Geometry check sheet. Reference: the model listing, model coordinates, mm. A direction names the side the tool comes from. Round coordinates to 2 decimals unless told otherwise and drop trailing zeros. Loops run counter-clockwise (first coordinate to the right, second up) from the corner with the lowest first, then second, coordinate; pieces in that order, holes last. Notation, with made-up numbers: M 71,52 L 75,52 A13 cw 75,63 Z; hole C 68,77 d10. An arc over 180 degrees is marked long. Write item = value, one per line.
from build123d import *

# Parameters (mm, degrees)
F0_R     = 3
F1_DEPTH = 5
F3_DEPTH = 115
F5_DEPTH = 25
F7_DEPTH = 25


with BuildPart() as f1:
    # F0 (on Top) → F1 (new body)
    with BuildSketch(Plane.XY):
        Polygon((-74.838845, -4.279941), (-74.838845, -104.279941), (35.161155, -104.279941), (35.161155, -4.279941), (30.161155, -4.279941), (30.161155, -39.279941), (-69.838845, -39.279941), (-69.838845, -4.279941), align=None)
        with Locations((-49.838845, -54.279941)):
            Circle(F0_R, mode=Mode.SUBTRACT)
        with Locations((10.161155, -54.279941)):
            Circle(F0_R, mode=Mode.SUBTRACT)
    extrude(amount=F1_DEPTH)

    # F2 (on face) → F3 (join)
    with BuildSketch(Plane.XY.offset(5)):
        Polygon((-74.838845, -104.279941), (-69.838845, -104.279941), (-69.838845, -39.279941), (-69.838845, -4.279941), (-74.838845, -4.279941), align=None)
        Polygon((30.161155, -39.279941), (30.161155, -104.279941), (35.161155, -104.279941), (35.161155, -4.279941), (30.161155, -4.279941), align=None)
    extrude(amount=F3_DEPTH)

    # F4 (on face) → F5 (cut)
    with BuildSketch(Plane.YZ.offset(35.161155)):
        Polygon((-104.279941, 30), (-34.279941, 120), (-104.279941, 120), align=None)
        with BuildLine():
            Line((-4.279941, 100), (-4.279941, 109.995835))
            Line((-4.279941, 109.995835), (-14.075894, 109.995835))
            Line((-14.075894, 109.995835), (-14.483987, 109.995835))
            ThreePointArc((-14.483987, 109.995835), (-19.2789, 104.897956), (-14.279941, 100))
            Line((-14.279941, 100), (-4.279941, 100))
        make_face()
    extrude(amount=-F5_DEPTH, mode=Mode.SUBTRACT)

    # F6 (on face) → F7 (cut)
    with BuildSketch(Plane(origin=(-74.838845, 0, 0), x_dir=(0, -1, 0), z_dir=(-1, 0, 0))):
        with BuildLine():
            Line((13.948806, 109.989023), (4.279941, 109.989023))
            Line((4.279941, 109.989023), (4.279941, 100))
            Line((4.279941, 100), (14.279941, 100))
            ThreePointArc((14.279941, 100), (19.277196, 104.834341), (14.611076, 109.989023))
            Line((14.611076, 109.989023), (13.948806, 109.989023))
        make_face()
        Polygon((104.279941, 120), (34.279941, 120), (104.279941, 30), align=None)
    extrude(amount=-F7_DEPTH, mode=Mode.SUBTRACT)


solid = f1.part
(1) Tool access check on faces 1 (the flat face through (33, -9, 109.996)), 2 (the flat face through (33, -4.28, 115)), 3 (the flat face through (-21, -71, 5)). Record the directions out of +Z, -Z, +X, -X, +Y, -Y that give a thin tool (end or side, any length) a straight path to the whole face; none if there is none.
Result set:
face_1 = +X, -X, +Y
face_2 = +Z, -Z, +X, -X, +Y
face_3 = +Z, +Y, -Y
(2) Depth check by flat-ended pin: pin 1 Ø19.5 at (x, y) = (0.5, -56.5) entering from +Z; pin 2 Ø2.5 at (x, z) = (-20.5, 2.5) entering from +Y; pin 3 Ø5.5 at (x, y) = (10.16, -54.28) entering from +Z. Enter the tip coordinate at first touch or a pass-through.
Result set:
pin_1 = 5
pin_2 = -39.28
pin_3 = through
(3) Sectioned sample at C-C on x = 18. Record the cut outline in (y, z).
Result set:
outline = M -104.28,0 L -39.28,0 L -39.28,5 L -104.28,5 Z
(4) Material ranges on line 1 along X through (y, z) = (-51, 51); line 2 along Z through (x, y) = (-2, -55), recorded low to high. Write a range as from..to.
Result set:
line_1 = -74.84..-69.84, 30.16..35.16
line_2 = 0..5
(5) Sectioned sample at D-D on y = -77. Record the cut outline in (x, z).
Result set:
outline = M -74.84,0 L 35.16,0 L 35.16,65.07 L 30.16,65.07 L 30.16,5 L -69.84,5 L -69.84,65.07 L -74.84,65.07 Z
(6) Release check for a two-part mould opening along X. For faces 4 (the cylindrical face through (9.51, -57.21, 2.46)), 5 (the flat face through (-72, -4.28, 115)), 6 (the flat face through (-19, -39.28, 2)), 7 (the flat face through (35.161, -44, 46)) record: released by +X, released by -X, zero draft, split by the parting line, or undercut.
Result set:
face_4 = undercut
face_5 = zero draft
face_6 = undercut
face_7 = released by +X
(7) Sectioned sample at A-A on y = -26.5. Record the cut outline in (x, z), then the cut area to 3 significant figures.
Result set:
outline = M -74.84,0 L -69.84,0 L -69.84,120 L -74.84,120 Z; M 30.16,0 L 35.16,0 L 35.16,120 L 30.16,120 Z
area = 1,200 mm2
(8) Sectioned sample at B-B on z = 16.5. Record the cut outline in (x, y).
Result set:
outline = M -74.84,-104.28 L -69.84,-104.28 L -69.84,-4.28 L -74.84,-4.28 Z; M 30.16,-104.28 L 35.16,-104.28 L 35.16,-4.28 L 30.16,-4.28 Z
